Geometry check sheet. Reference: the model listing, model coordinates, mm. A direction names the side the tool comes from. Coordinates: 2 decimals unless noted, no trailing zeros. Write each loop counter-clockwise with the first axis right and the second up, starting at its lowest first coordinate (ties: lowest second). Pieces come first, ordered by that corner, then holes. Notation, with made-up numbers: M 29.5,19 L 81.5,19 A16 cw 81.5,25 Z; hole C 30.25,11 d1. An arc over 180 degrees is marked long. Answer as a JSON object with one key per item and string values. Group by question number.
```python
from build123d import *

# Parameters (mm, degrees)
F0_R     = 1.05
F0_R_2   = 1.5
F1_DEPTH = 1.5
F3_R     = 1.2
F4_R     = 1.95
F4_R_2   = 1.05
F5_DEPTH = 5
F4_R_3   = 2.4
F4_R_4   = 1.5
F6_DEPTH = 7


with BuildPart() as f1:
    # F0 (on Top) → F1 (new body)
    with BuildSketch(Plane.XY):
        Polygon((37, 30.5212866254), (-37, 30.5212866254), (-37, 4.6800224319), (-37, -1.3199775681), (-37, -29.3157063685), (37, -29.3157063685), (37, -1.3199775681), (37, 4.6800224319), align=None)
        with Locations((-29, -22.5189467669)):
            Circle(F0_R, mode=Mode.SUBTRACT)
        with Locations((-29, 0.4810532331)):
            Circle(F0_R, mode=Mode.SUBTRACT)
        with Locations((29, -22.5189467669)):
            Circle(F0_R, mode=Mode.SUBTRACT)
        with Locations((29, 0.4810532331)):
            Circle(F0_R, mode=Mode.SUBTRACT)
        with Locations((-15.2, 24.5643973112)):
            Circle(F0_R_2, mode=Mode.SUBTRACT)
        with Locations((15.2, 8.3643973112)):
            Circle(F0_R_2, mode=Mode.SUBTRACT)
        with BuildLine():
            Line((-37, -1.3199775681), (-37, 4.6800224319))
            Line((-37, 4.6800224319), (-42, 4.6800224319))
            ThreePointArc((-42, 4.6800224319), (-43.4142135624, 4.0942359942), (-44, 2.6800224319))
            Line((-44, 2.6800224319), (-44, 0.6800224319))
            ThreePointArc((-44, 0.6800224319), (-43.4142135624, -0.7341911305), (-42, -1.3199775681))
            Line((-42, -1.3199775681), (-37, -1.3199775681))
        make_face()
        with Locations((-41, 1.6800224319)):
            Circle(F0_R_2, mode=Mode.SUBTRACT)
        with BuildLine():
            Line((42, 4.6800224319), (37, 4.6800224319))
            Line((37, 4.6800224319), (37, -1.3199775681))
            Line((37, -1.3199775681), (42, -1.3199775681))
            ThreePointArc((42, -1.3199775681), (43.4142135624, -0.7341911305), (44, 0.6800224319))
            Line((44, 0.6800224319), (44, 2.6800224319))
            ThreePointArc((44, 2.6800224319), (43.4142135624, 4.0942359942), (42, 4.6800224319))
        make_face()
        with Locations((41, 1.6800224319)):
            Circle(F0_R_2, mode=Mode.SUBTRACT)
    extrude(amount=-F1_DEPTH)

    # F3
    f3_edges = [f1.edges().sort_by_distance(p)[0] for p in [
        (-37, -1.319978, -0.75),
        (-37, 4.680022, -0.75),
        (37, -1.319978, -0.75),
        (37, 4.680022, -0.75),
    ]]
    fillet(f3_edges, radius=F3_R)

    # F4 (on face) → F5 (join)
    with BuildSketch(Plane.XY):
        with Locations((-29, 0.4810532331)):
            Circle(F4_R)
        with Locations((-29, 0.4810532331)):
            Circle(F4_R_2, mode=Mode.SUBTRACT)
        with Locations((-29, -22.5189467669)):
            Circle(F4_R)
        with Locations((-29, -22.5189467669)):
            Circle(F4_R_2, mode=Mode.SUBTRACT)
        with Locations((29, -22.5189467669)):
            Circle(F4_R)
        with Locations((29, -22.5189467669)):
            Circle(F4_R_2, mode=Mode.SUBTRACT)
        with Locations((29, 0.4810532331)):
            Circle(F4_R)
        with Locations((29, 0.4810532331)):
            Circle(F4_R_2, mode=Mode.SUBTRACT)
    extrude(amount=F5_DEPTH)

    # F4 (on face) → F6 (join)
    with BuildSketch(Plane.XY):
        with Locations((-15.2, 24.5643973112)):
            Circle(F4_R_3)
        with Locations((-15.2, 24.5643973112)):
            Circle(F4_R_4, mode=Mode.SUBTRACT)
        with Locations((15.2, 8.3643973112)):
            Circle(F4_R_3)
        with Locations((15.2, 8.3643973112)):
            Circle(F4_R_4, mode=Mode.SUBTRACT)
    extrude(amount=F6_DEPTH)


solid = f1.part
```
1) Go/stop test with flat-tipped pins: pin 1 Ø1.6 at (x, z) = (40, -1) entering from -Y; pin 2 Ø1.6 at (y, z) = (18, -1) entering from +X; pin 3 Ø4 at (x, y) = (-15.2, 24.56) entering from +Z; pin 4 Ø1 at (y, z) = (1.5, 2) entering from -X. Record where each tip stops, or that it passes through.
2) Section check C-C (z = 1.25). State how many separate pieces and enclosed holes the cut face has, then the cut area to 3 significant figures.
3) Draft check along X on faces 1 (the cylindrical face through (29.9, -24.25, 2.46)), 2 (the flat face through (-27.7, 0.5, 5)), 3 (the cylindrical face through (-15.72, 22.22, 3.45)). Enter one of: +X half, -X half, draft (parallel to the pull), parting line (faces both ways), or undercut.
4) Material ranges on probe 1 along Y at (x, z) = (29, 4); probe 2 along Y at (x, z) = (-29, -1.15); probe 3 along X at (y, z) = (-22, 1.5), recorded low to high. Write a range as [from, to].
5) Section check B-B (x = 41). Record the cut outline in (y, z), then the cut area to 3 significant figures.
6) Section check D-D (y = 13). Record the cut outline in (x, z), then the cut area to 3 significant figures.
7) Section check A-A (x = -29). Record the cut outline in (y, z).
8) Set-up check for faces 4 (the cylindrical face through (-43.43, -0.72, -0.74)), 5 (the cylindrical face through (-27.2, -0.27, 2.46)): record each of +Z, -Z, +X, -X, +Y, -Y from which the full face is reachable in a straight line by a thin tool's end or side.
Entries:
{
 "1": {"pin 1": "y = -1.32", "pin 2": "x = 37", "pin 3": "z = 7", "pin 4": "x = -30.88"},
 "2": {"separate pieces": "6", "enclosed holes": "6", "area": "56.0 mm^2"},
 "3": {"face 1": "undercut", "face 2": "draft", "face 3": "parting line"},
 "4": {"probe 1": "[-24.47, -23.57], [-21.47, -20.57], [-1.47, -0.57], [1.53, 2.43]", "probe 2": "[-29.32, -23.57], [-21.47, -0.57], [1.53, 30.52]", "probe 3": "[-30.88, -29.91], [-28.09, -27.12], [27.12, 28.09], [29.91, 30.88]"},
 "5": {"outline": "M -1.32,-1.5 L 0.18,-1.5 L 0.18,0 L -1.32,0 Z; M 3.18,-1.5 L 4.68,-1.5 L 4.68,0 L 3.18,0 Z", "area": "4.50 mm^2"},
 "6": {"outline": "M -37,-1.5 L 37,-1.5 L 37,0 L -37,0 Z", "area": "111 mm^2"},
 "7": {"outline": "M -29.32,-1.5 L -23.57,-1.5 L -23.57,5 L -24.47,5 L -24.47,0 L -29.32,0 Z; M -21.47,-1.5 L -0.57,-1.5 L -0.57,5 L -1.47,5 L -1.47,0 L -20.57,0 L -20.57,5 L -21.47,5 Z; M 1.53,-1.5 L 30.52,-1.5 L 30.52,0 L 2.43,0 L 2.43,5 L 1.53,5 Z"},
 "8": {"face 4": "+Z, -Z, -X, -Y", "face 5": "+Z"}
}
